The model under review builds one solid part; all positions refer to its coordinate system, in mm. A direction names the side the tool comes from. Round coordinates to 2 decimals unless told otherwise and drop trailing zeros. Loops run counter-clockwise (first coordinate to the right, second up) from the corner with the lowest first, then second, coordinate; pieces in that order, holes last. Notation, with made-up numbers: (36, -28) -> (65, -28) arc R18 cw to (65, 2) -> close; hole circle Ø11 at (23, 66.5). An arc over 180 degrees is marked (long way). Write each question's results on one line, items separated by ' | '. Start each with the question number.
Item 1: We need section B-B (y = 13.75). Give the boundary of the cut face in (x, z), and give its area (3 significant figures).
Item 2: Mouldability with a two-part tool opening along X and no side actions: class faces 1 (the cylindrical face through (-0.234, -11.965, 10.97)), 2 (the flat face through (-1, -27, 3)), 3 (the flat face through (-44.5, 1, 4)) as pulls with the +X half, pulls with the -X half, needs draft (parallel to the pull), parting line crosses it, or undercut.
Item 3: Clearance check with flat-ended pins moving along their axes: pin 1 Ø2 at (x, z) = (-16.5, 7.5) entering from +Y; pin 2 Ø3 at (x, z) = (-16, 3.5) entering from +Y; pin 3 Ø2.5 at (x, z) = (12, 0.5) entering from -Y. State where each tip first meets the part, or that it passes through.
Item 4: For L1, parallel to X at y = 32.25, z = 5.9 (3 decimals); L2, parallel to Z at x = 32.5, y = 27; L3, parallel to X at y = 11.5, z = 0.25, list the stretches that pass through material, from the lowest coordinate up. Write a range as from..to.
Item 5: We need section A-A (y = -9). Give the boundary of the cut face in (x, z), and give its area (3 significant figures).
Item 6: We need section C-C (x = -33). Give the boundary of the cut face in (y, z), and give its area (3 significant figures).
Item 7: Tool access review of faces 4 (the flat face through (-1, -30, 8)), 5 (the flat face through (2, 15, 9.5)), 6 (the flat face through (-3, 25, 8.4)): name each direction out of +Z, -Z, +X, -X, +Y, -Y from which nothing blocks a thin tool from reaching the whole face with its end or side.
Item 8: We need section D-D (x = 36). Give the boundary of the cut face in (y, z).
from build123d import *

# Parameters (mm, degrees)
BOSS_EXTRUDE1_DEPTH            = 6.4
SKETCH2_W                      = 89
SKETCH2_H                      = 70
BOSS_EXTRUDE2_DEPTH            = 2
SKETCH3_W                      = 8
SKETCH3_H                      = 6
CUT_EXTRUDE1_DEPTH             = 2
SKETCH5_W                      = 89
SKETCH5_H                      = 70
BOSS_EXTRUDE3_DEPTH            = 6
CBORE_FOR_M3_SHCS1_D           = 3.6
CBORE_FOR_M3_SHCS1_CBORE_D     = 7
CBORE_FOR_M3_SHCS1_CBORE_DEPTH = 11.5
SKETCH8_W                      = 9.5
SKETCH8_H                      = 4.5
CUT_EXTRUDE3_DEPTH             = 6
SKETCH10_W                     = 33.5
SKETCH10_H                     = 5
CUT_EXTRUDE4_DEPTH             = 2
M2_5X0_45_TAPPED_HOLE1_D       = 2.05
M2_5X0_45_TAPPED_HOLE1_DEPTH   = 7.25
M2_5X0_45_TAPPED_HOLE1_TIP     = 0.615882135
CUT_EXTRUDE5_DEPTH             = 97.43526326
FILLET1_R                      = 3


with BuildPart() as part:
    # Sketch1 → Boss-Extrude1 (new body)
    with BuildSketch(Plane.XY):
        Polygon((-38.5, -15), (-38.5, 35), (-44.5, 35), (-44.5, -35), (44.5, -35), (44.5, 35), (41.5, 35), (41.5, -15), align=None)
    extrude(amount=BOSS_EXTRUDE1_DEPTH)

    # Sketch2 → Boss-Extrude2 (add)
    with BuildSketch(Plane(origin=(0, 0, 0), x_dir=(-1, 0, 0), z_dir=(0, 0, -1))):
        Rectangle(SKETCH2_W, SKETCH2_H)
    extrude(amount=BOSS_EXTRUDE2_DEPTH)

    # Sketch3 → Cut-Extrude1 (cut)
    with BuildSketch(Plane.XY):
        with Locations((-32.5, 32)):
            Rectangle(SKETCH3_W, SKETCH3_H)
    extrude(amount=-CUT_EXTRUDE1_DEPTH, mode=Mode.SUBTRACT)

    # Sketch5 → Boss-Extrude3 (add)
    with BuildSketch(Plane.XY.offset(6.4)):
        Rectangle(SKETCH5_W, SKETCH5_H)
    extrude(amount=BOSS_EXTRUDE3_DEPTH)

    # CBORE for M3 SHCS1 (through all)
    with Locations(Plane(origin=(0, 0, -2), x_dir=(-1, 0, 0), z_dir=(0, 0, -1))):
        with Locations((0, -13.75), (0, 13.75), (-13.75, 0), (13.75, 0)):
            CounterBoreHole(CBORE_FOR_M3_SHCS1_D / 2, CBORE_FOR_M3_SHCS1_CBORE_D / 2, CBORE_FOR_M3_SHCS1_CBORE_DEPTH)

    # Sketch8 → Cut-Extrude3 (cut)
    with BuildSketch(Plane.XY.offset(12.4)):
        with Locations((5.25, 7.75)):
            Rectangle(SKETCH8_W, SKETCH8_H)
    extrude(amount=-CUT_EXTRUDE3_DEPTH, mode=Mode.SUBTRACT)

    # Sketch10 → Cut-Extrude4 (cut)
    with BuildSketch(Plane(origin=(0, 0, 6.4), x_dir=(-1, 0, 0), z_dir=(0, 0, -1))):
        Polygon((-10, 35), (-10, 10), (5, 10), (5, 30), (5, 35), align=None)
        with Locations((21.75, 32.5)):
            Rectangle(SKETCH10_W, SKETCH10_H)
    extrude(amount=-CUT_EXTRUDE4_DEPTH, mode=Mode.SUBTRACT)

    # M2.5x0.45 Tapped Hole1
    with Locations(Plane(origin=(0, 35, 0), x_dir=(1, 0, 0), z_dir=(0, 1, 0))):
        with Locations((-41.5, -5.9), (41.5, -9.4), (15.5, -9.4)):
            Hole(M2_5X0_45_TAPPED_HOLE1_D / 2, depth=M2_5X0_45_TAPPED_HOLE1_DEPTH)
            with Locations((0, 0, -(M2_5X0_45_TAPPED_HOLE1_DEPTH + M2_5X0_45_TAPPED_HOLE1_TIP / 2))):  # 118° drill point
                Cone(0, M2_5X0_45_TAPPED_HOLE1_D / 2, M2_5X0_45_TAPPED_HOLE1_TIP, mode=Mode.SUBTRACT)

    # Sketch13 → Cut-Extrude5 (cut, through all)
    with BuildSketch(Plane.ZY.offset(44.5)):
        Polygon((-2, -35), (8, -35), (8, -25), (3, -25), (3, -30), (-2, -30), align=None)
    extrude(amount=-CUT_EXTRUDE5_DEPTH, mode=Mode.SUBTRACT)

    # Fillet1
    fillet1_edges = [part.edges().sort_by_distance(p)[0] for p in [
        (44.5, -35, 10.2),
        (-44.5, -35, 10.2),
        (-44.5, 0, 12.4),
        (0, -35, 12.4),
        (44.5, 0, 12.4),
    ]]
    fillet(fillet1_edges, radius=FILLET1_R)


solid = part.part
Here are the results:
1) outline: (-44.5, -2) -> (-3.5, -2) -> (-3.5, 0) -> (-38.5, 0) -> (-38.5, 6.4) -> (-5, 6.4) -> (-5, 8.4) -> (-3.5, 8.4) -> (-3.5, 9.5) -> (-1.8, 9.5) -> (-1.8, 12.4) -> (-41.5, 12.4) arc R3 ccw to (-44.5, 9.4) -> close; (1.8, 9.5) -> (3.5, 9.5) -> (3.5, 8.4) -> (10, 8.4) -> (10, 6.4) -> (41.5, 6.4) -> (41.5, 0) -> (3.5, 0) -> (3.5, -2) -> (44.5, -2) -> (44.5, 9.4) arc R3 ccw to (41.5, 12.4) -> (1.8, 12.4) -> close | area: 704 mm2
2) face 1: undercut | face 2: needs draft | face 3: pulls with the -X half
3) pin 1: stops at y = 35 | pin 2: stops at y = -15 | pin 3: stops at y = -30
4) L1: x = -44.5..-42.525, -40.475..-38.5, 41.5..44.5 | L2: z = -2..0, 6.4..12.4 | L3: x = -44.5..-38.5, 41.5..44.5
5) outline: (-44.5, -2) -> (44.5, -2) -> (44.5, 9.4) arc R3 ccw to (41.5, 12.4) -> (-41.5, 12.4) arc R3 ccw to (-44.5, 9.4) -> close; hole (-38.5, 0) -> (41.5, 0) -> (41.5, 6.4) -> (-38.5, 6.4) -> close | area: 766 mm2
6) outline: (-35, 8) -> (-25, 8) -> (-25, 3) -> (-30, 3) -> (-30, -2) -> (29, -2) -> (29, 0) -> (-15, 0) -> (-15, 6.4) -> (30, 6.4) -> (30, 8.4) -> (35, 8.4) -> (35, 12.4) -> (-32, 12.4) arc R3 ccw to (-35, 9.4) -> close | area: 589 mm2
7) face 4: +X, -X, -Y | face 5: -Z | face 6: +Y
8) outline: (-35, 8) -> (-25, 8) -> (-25, 3) -> (-30, 3) -> (-30, -2) -> (35, -2) -> (35, 0) -> (-15, 0) -> (-15, 6.4) -> (35, 6.4) -> (35, 12.4) -> (-32, 12.4) arc R3 ccw to (-35, 9.4) -> close
